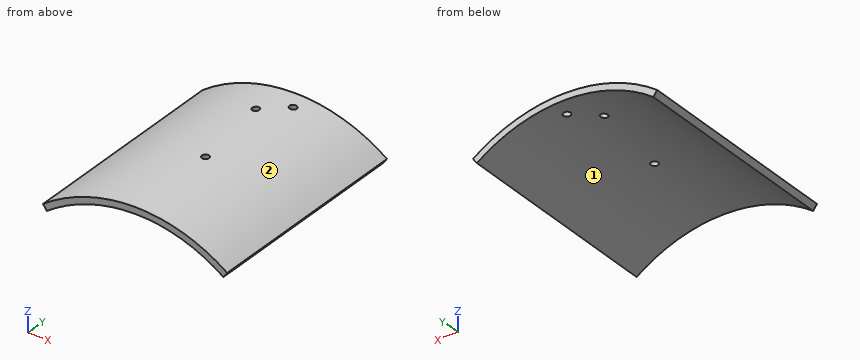
```python
from build123d import *

# Parameters (mm, degrees)
BOSS_EXTRUDE1_DEPTH = 114.3
SKETCH2_R           = 1.7526
CUT_EXTRUDE1_DEPTH  = 25.4
SKETCH3_W           = 89.096923456
SKETCH3_H           = 11.672787919
CUT_EXTRUDE2_DEPTH  = 25.4


with BuildPart() as part:
    # Sketch1 → Boss-Extrude1 (new body)
    with BuildSketch(Plane(origin=(0, 0, 0), x_dir=(1, 0, 0), z_dir=(0, 1, 0))):
        with BuildLine():
            Line((-42.692275823, -59.245423537), (-44.548461728, -61.821311517))
            ThreePointArc((-44.548461728, -61.821311517), (0, -76.2), (44.548461728, -61.821311517))
            Line((44.548461728, -61.821311517), (42.692275823, -59.245423537))
            ThreePointArc((42.692275823, -59.245423537), (0, -73.025), (-42.692275823, -59.245423537))
        make_face()
    extrude(amount=BOSS_EXTRUDE1_DEPTH)

    # Sketch2 → Cut-Extrude1 (cut)
    with BuildSketch(Plane(origin=(0, 0, 59.245423537), x_dir=(-1, 0, 0), z_dir=(0, 0, -1))):
        with Locations((0, 54.61)):
            Circle(SKETCH2_R)
        with Locations((-5.55625, 105.41)):
            Circle(SKETCH2_R)
        with Locations((5.55625, 95.885)):
            Circle(SKETCH2_R)
    extrude(amount=-CUT_EXTRUDE1_DEPTH, mode=Mode.SUBTRACT)

    # Sketch3 → Cut-Extrude2 (cut)
    with BuildSketch(Plane(origin=(0, 0, 59.245423537), x_dir=(-1, 0, 0), z_dir=(0, 0, -1))):
        with Locations((0, 1.783606041)):
            Rectangle(SKETCH3_W, SKETCH3_H)
    extrude(amount=-CUT_EXTRUDE2_DEPTH, mode=Mode.SUBTRACT)


solid = part.part
```
Can you work these out from the model? Positions are in its coordinate system, mm. Face numbers are marked on the shaded views. Give positions to 0.01 mm unless a question says otherwise; leave off trailing zeros. Loops run counter-clockwise (first coordinate to the right, second up) from the corner with the lowest first, then second, coordinate; pieces in that order, holes last. Notation, with made-up numbers: M 55,20 L 97,20 A25 ccw 97,32 Z; hole C 41,77 d9. An arc over 180 degrees is marked long. Use CSV: the item, a comma, the result in double quotes. Start each with the question number.
1. Imagine slicing it at B-B, the plane z = 64. Write out the boundary of the cut face in (x, y), plus the area to 3 significant figures.
2. Imagine slicing it at C-C, the plane x = -11.5. Write out the boundary of the cut face in (y, z).
3. Imagine slicing it at A-A, the plane x = 0. Write out the boundary of the cut face in (y, z) (3 decimals), plus the area to 3 significant figures.
4. If we mould it in two halves opening along X, with no side actions, what happens to the marked faces 1 and 2? For each: released by +X, released by -X, zero draft, split by the parting line, or undercut.
5. If I drill on L1, parallel to Y at x = 0, z = 75.5; L2, parallel to X at y = 76, z = 67.5; L3, parallel to X at y = 93.5, z = 60.75, over which ranges is the centre line in solid material (lowest first)?
6. Imagine slicing it at D-D, the plane x = 24. Write out the boundary of the cut face in (y, z), plus the area to 3 significant figures.
7. For P1, Ø2, axis at y = 66.5, z = 69, coming from the -X side; P2, Ø6, axis at x = 17, y = 29.5, coming from the +Z side; P3, Ø10, axis at y = 27.5, z = 62.5, coming from the -X side, each with a flat end and sliding along its axis, tell me the tip position at first contact or that it passes through.
Response values:
1,outline,"M -41.36,7.62 L -35.17,7.62 L -35.17,114.3 L -41.36,114.3 Z; M 35.17,7.62 L 41.36,7.62 L 41.36,114.3 L 35.17,114.3 Z"
1,area,"1,320 mm^2"
2,outline,"M 7.62,72.11 L 114.3,72.11 L 114.3,75.33 L 7.62,75.33 Z"
3,outline,"M 7.62,73.025 L 52.857,73.025 L 52.857,76.2 L 7.62,76.2 Z; M 56.363,73.025 L 114.3,73.025 L 114.3,76.2 L 56.363,76.2 Z"
3,area,"328 mm^2"
4,face 1,"undercut"
4,face 2,"split by the parting line"
5,L1,"7.62 to 52.86, 56.36 to 114.3"
5,L2,"-35.36 to -27.86, 27.86 to 35.36"
5,L3,"-43.78 to -40.52, 40.52 to 43.78"
6,outline,"M 7.62,68.97 L 114.3,68.97 L 114.3,72.32 L 7.62,72.32 Z"
6,area,"358 mm^2"
7,P1,"x = -34.39"
7,P2,"z = 74.9"
7,P3,"x = -44.55"
